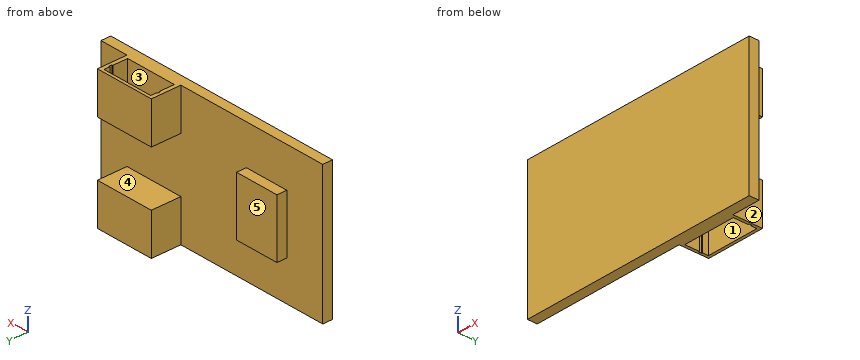
```python
from build123d import *

# Parameters (mm, degrees)
SKETCH1_W           = 24.7
SKETCH1_H           = 13.9
BOSS_EXTRUDE1_DEPTH = 1
SKETCH2_W           = 6
SKETCH2_H           = 4.2
BOSS_EXTRUDE2_DEPTH = 3
CUT_EXTRUDE1_DEPTH  = 3
CUT_EXTRUDE2_DEPTH  = 3
SKETCH6_W           = 4.5
SKETCH6_H           = 5.9
BOSS_EXTRUDE3_DEPTH = 1


with BuildPart() as part:
    # Sketch1 → Boss-Extrude1 (new body)
    with BuildSketch(Plane(origin=(0, 0, 0), x_dir=(1, 0, 0), z_dir=(0, 1, 0))):
        Rectangle(SKETCH1_W, SKETCH1_H)
    extrude(amount=BOSS_EXTRUDE1_DEPTH)

    # Sketch2 → Boss-Extrude2 (add)
    with BuildSketch(Plane(origin=(0, 1, 0), x_dir=(1, 0, 0), z_dir=(0, 1, 0))):
        with Locations((6.45, -4.85)):
            Rectangle(SKETCH2_W, SKETCH2_H)
        with Locations((6.45, 4.85)):
            Rectangle(SKETCH2_W, SKETCH2_H)
    extrude(amount=BOSS_EXTRUDE2_DEPTH)

    # Sketch3 → Cut-Extrude1 (cut)
    with BuildSketch(Plane.XY.offset(6.95)):
        Polygon((3.85, 3.7), (3.85, 3.1), (3.75, 3.1), (3.75, 2.8), (3.85, 2.8), (3.85, 1.3), (9.05, 1.3), (9.05, 2.8), (9.15, 2.8), (9.15, 3.1), (9.05, 3.1), (9.05, 3.7), align=None)
    extrude(amount=-CUT_EXTRUDE1_DEPTH, mode=Mode.SUBTRACT)

    # Sketch5 → Cut-Extrude2 (cut)
    with BuildSketch(Plane(origin=(0, 0, -6.95), x_dir=(-1, 0, 0), z_dir=(0, 0, -1))):
        Polygon((-9.15, 3.7), (-9.15, 3.1), (-9.25, 3.1), (-9.25, 2.8), (-9.15, 2.8), (-9.15, 1.3), (-3.75, 1.3), (-3.75, 2.8), (-3.65, 2.8), (-3.65, 3.1), (-3.75, 3.1), (-3.75, 3.7), align=None)
    extrude(amount=-CUT_EXTRUDE2_DEPTH, mode=Mode.SUBTRACT)

    # Sketch6 → Boss-Extrude3 (add)
    with BuildSketch(Plane(origin=(0, 1, 0), x_dir=(1, 0, 0), z_dir=(0, 1, 0))):
        with Locations((-6.1, 0)):
            Rectangle(SKETCH6_W, SKETCH6_H)
    extrude(amount=BOSS_EXTRUDE3_DEPTH)


solid = part.part
```
For this review, take the finished solid that the model builds, in its own axes (mm). Face numbers are marked on the shaded views. A direction names the side the tool comes from. Coordinates: 2 decimals unless noted, no trailing zeros. Write each loop counter-clockwise with the first axis right and the second up, starting at its lowest first coordinate (ties: lowest second). Pieces come first, ordered by that corner, then holes. Notation, with made-up numbers: (11, 64.25) -> (35, 64.25) arc R13 ccw to (35, 69.25) -> close; hole circle Ø5 at (35.5, 43). An arc over 180 degrees is marked (long way). Put each result on its own line as item: value.
Q1. Take a section at B-B, the plane z = -5. State the section outline as (x, y) points, then the cut area to 3 significant figures.
From the geometry:
outline: (-12.35, 0) -> (12.35, 0) -> (12.35, 1) -> (9.45, 1) -> (9.45, 4) -> (3.45, 4) -> (3.45, 1) -> (-12.35, 1) -> close; hole (3.65, 2.8) -> (3.75, 2.8) -> (3.75, 1.3) -> (9.15, 1.3) -> (9.15, 2.8) -> (9.25, 2.8) -> (9.25, 3.1) -> (9.15, 3.1) -> (9.15, 3.7) -> (3.75, 3.7) -> (3.75, 3.1) -> (3.65, 3.1) -> close
area: 29.7 mm2
Q2. Take a section at A-A, the plane y = 2.5. State the section outline as (x, z) points, then the cut area to 3 significant figures.
From the geometry:
outline: (3.45, -6.95) -> (3.75, -6.95) -> (3.75, -3.95) -> (9.15, -3.95) -> (9.15, -6.95) -> (9.45, -6.95) -> (9.45, -2.75) -> (3.45, -2.75) -> close; (3.45, 2.75) -> (9.45, 2.75) -> (9.45, 6.95) -> (9.05, 6.95) -> (9.05, 3.95) -> (3.85, 3.95) -> (3.85, 6.95) -> (3.45, 6.95) -> close
area: 18.6 mm2
Q3. Take a section at D-D, the plane z = 1.5. State the section outline as (x, y) points.
From the geometry:
outline: (-12.35, 0) -> (12.35, 0) -> (12.35, 1) -> (-3.85, 1) -> (-3.85, 2) -> (-8.35, 2) -> (-8.35, 1) -> (-12.35, 1) -> close
Q4. Tool access review of the marked faces 1, 2 and 3: name each direction out of +Z, -Z, +X, -X, +Y, -Y from which nothing blocks a thin tool from reaching the whole face with its end or side.
From the geometry:
face 1: -Z
face 2: +Z, -Z, +X, +Y
face 3: +Z
Q5. The part is to be moulded in two halves that separate along Z. For the marked faces 4 and 5, say which applies: +Z half, -Z half, draft (parallel to the pull), parting line (faces both ways), or undercut.
From the geometry:
face 4: undercut
face 5: draft
Q6. Wall thickness on L1, parallel to X at y = 3.4, z = -4.5; L2, parallel to Y at x = 4.5, z = 4.75; L3, parallel to X at y = 1.8, z = 4: over which ranges is each line inside the solid? List them lowest first.
From the geometry:
L1: x = 3.45 to 3.75, 9.15 to 9.45
L2: y = 0 to 1.3, 3.7 to 4
L3: x = 3.45 to 3.85, 9.05 to 9.45
Q7. Clearance check with flat-ended pins moving along their axes: pin 1 Ø1.2 at (y, z) = (2, -6) entering from +X; pin 2 Ø5 at (x, z) = (-2, -4) entering from +Y; pin 3 Ø2 at (y, z) = (2.5, 5) entering from -X; pin 4 Ø1.5 at (x, z) = (9, -4.5) entering from -Y. State where each tip first meets the part, or that it passes through.
From the geometry:
pin 1: stops at x = 9.45
pin 2: stops at y = 2
pin 3: stops at x = 3.45
pin 4: stops at y = 0
Q8. Take a section at C-C, the plane x = -5.25. State the section outline as (y, z) points, then the cut area to 3 significant figures.
From the geometry:
outline: (0, -6.95) -> (1, -6.95) -> (1, -2.95) -> (2, -2.95) -> (2, 2.95) -> (1, 2.95) -> (1, 6.95) -> (0, 6.95) -> close
area: 19.8 mm2
